Job drawing, mm, ordinate dimensions from the low corner. One solid piece. Round coordinates to 2 decimals unless told otherwise and drop trailing zeros. Loops run counter-clockwise (first coordinate to the right, second up) from the corner with the lowest first, then second, coordinate; pieces in that order, holes last.
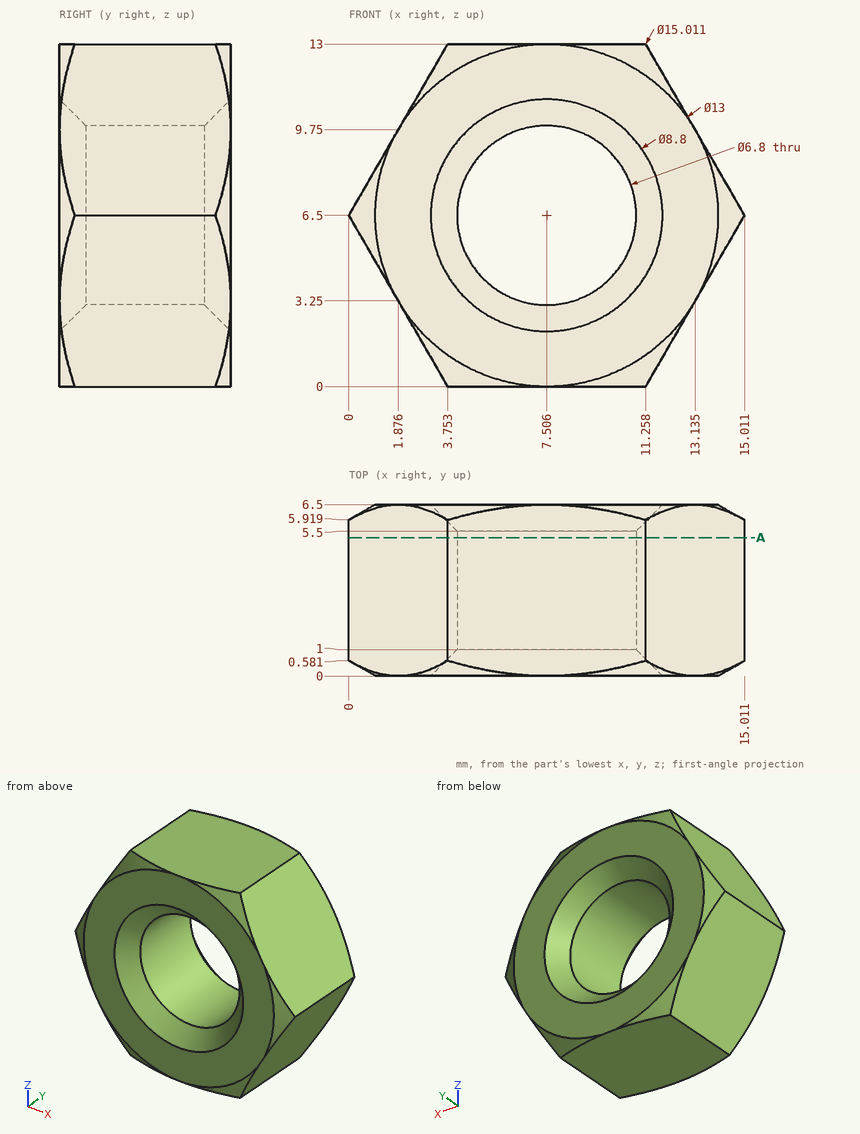
1) Wall check: line 1 along X through (y, z) = (1.5, 4) (1 decimal); line 2 along X through (y, z) = (2.25, 5.75); line 3 along Y through (x, z) = (11.25, 5.75). Give the ranges that are in metal, low to high.
Values:
line 1: x = 1.4 to 5.2, 9.8 to 13.6
line 2: x = 0.43 to 4.19, 10.82 to 14.58
line 3: y = 0.58 to 5.92
2) Slice it at A-A, the plane y = 5.25. Give the cut face in (x, z) (1 decimal), then the cut area to 3 significant figures.
Values:
outline: (0, 6.5) - (3.8, 0) - (11.3, 0) - (15, 6.5) - (11.3, 13) - (3.8, 13) - close; hole circle Ø6.8 at (7.5, 6.5)
area: 110 mm2
3) Drop a flat-ended pin along its axis: pin 1 Ø1 at (y, z) = (5, 9) entering from -X (1 decimal). Give the stop position or say it passes through.
Values:
pin 1: stops at x = 1.2
